from build123d import *

# Parameters (mm, degrees)
SKETCH1_R                    = 1.8288
BASE_FLANGE1_DEPTH           = 1.5875
EDGE_FLANGE2_STRIP_W         = 7.8232
EDGE_FLANGE2_STRIP_H         = 1.5875
EDGE_FLANGE2_STRIP_CUT_DEPTH = 6.35
EDGE_FLANGE2_DEPTH           = 6.35
SKETCH19_W                   = 5.65
SKETCH19_H                   = 12
TAB1_DEPTH                   = 1.5875
HOLE1_START                  = -28.75
HOLE1_OUTLINE_R              = 1.8288
HOLE1_DEPTH                  = 1.5875
FILLET1_R                    = 6


# Read off the part's stored shape, not the designer's step: Hole1
# Sheet-metal steps are written as plain solids
with BuildPart() as part:
    # Sketch1 → Base-Flange1 (new body)
    with BuildSketch(Plane(origin=(0, 0, 0), x_dir=(1, 0, 0), z_dir=(0, 1, 0))):
        with BuildLine():
            Line((-25.575, 0), (-25.575, 6.35))
            Line((-25.575, 6.35), (-27.1625, 6.35))
            Line((-27.1625, 6.35), (-27.1625, 12.7))
            Line((-27.1625, 12.7), (0, 12.7))
            Line((0, 12.7), (25.575, 12.7))
            Line((25.575, 12.7), (25.575, 0))
            ThreePointArc((25.575, 0), (22.4, -3.175), (19.225, 0))
            Line((19.225, 0), (19.225, 6.35))
            Line((19.225, 6.35), (3.175, 6.35))
            Line((3.175, 6.35), (3.175, 0))
            ThreePointArc((3.175, 0), (0, -3.175), (-3.175, 0))
            Line((-3.175, 0), (-3.175, 6.35))
            Line((-3.175, 6.35), (-19.225, 6.35))
            Line((-19.225, 6.35), (-19.225, 0))
            ThreePointArc((-19.225, 0), (-22.4, -3.175), (-25.575, 0))
        make_face()
        with Locations(Location((0, 0, 0), (0, 0, 270))):
            Circle(SKETCH1_R, mode=Mode.SUBTRACT)
        with Locations(Location((22.4, 0, 0), (0, 0, 270))):
            Circle(SKETCH1_R, mode=Mode.SUBTRACT)
        with Locations(Location((-22.4, 0, 0), (0, 0, 270))):
            Circle(SKETCH1_R, mode=Mode.SUBTRACT)
    extrude(amount=BASE_FLANGE1_DEPTH)

    # Edge-Flange2 strip (across the edge) → Edge-Flange2 strip cut (cut)
    with BuildSketch(Plane(origin=(-27.1625, 1.5875, -12.7), x_dir=(1, 0, 0), z_dir=(0, 0, 1))):
        with Locations((-3.175, -0.79375)):
            Rectangle(EDGE_FLANGE2_STRIP_W, EDGE_FLANGE2_STRIP_H)
    extrude(amount=EDGE_FLANGE2_STRIP_CUT_DEPTH, mode=Mode.SUBTRACT)

    # Edge-Flange2 section (across the edge) → Edge-Flange2 (add)
    with BuildSketch(Plane(origin=(-27.1625, 1.5875, -12.7), x_dir=(1, 0, 0), z_dir=(0, 0, 1))):
        with BuildLine():
            Line((-1.5875, 0.7366), (-1.5875, 31.688))
            Line((-1.5875, 31.688), (0, 31.688))
            Line((0, 31.688), (0, 0.7366))
            ThreePointArc((0, 0.7366), (0.215745145, 0.215745145), (0.7366, 0))
            Line((0.7366, 0), (0.7366, -1.5875))
            ThreePointArc((0.7366, -1.5875), (-0.90678687, -0.90678687), (-1.5875, 0.7366))
        make_face()
    extrude(amount=EDGE_FLANGE2_DEPTH)

    # Sketch19 → Tab1 (add)
    with BuildSketch(Plane.ZY.offset(28.75)):
        with Locations((-3.525, 27.2755)):
            Rectangle(SKETCH19_W, SKETCH19_H)
    extrude(amount=-TAB1_DEPTH)

    # Hole1 outline → Hole1 (cut)
    with BuildSketch(Plane.YZ.offset(HOLE1_START)):
        with Locations((26.9255, -6.7)):
            Circle(HOLE1_OUTLINE_R)
    extrude(amount=HOLE1_DEPTH, mode=Mode.SUBTRACT)

    # Fillet1
    # the kernel refuses this fillet: 6 mm, written as the material it takes off along each edge
    with BuildSketch(Plane(origin=(-43.724457419, 21.2755, -0.7), x_dir=(0, 0, -1), z_dir=(1, 0, 0))) as fillet1_piece_1:
        with BuildLine():
            CenterArc((6, 5.989782968), FILLET1_R, 180, 86.655847796)
            Line((0, 5.989782968), (-0.12, 5.989782968))
            Line((-0.12, 5.989782968), (-0.12, 0))
            Line((-0.12, 0), (0, -0.12))
            ThreePointArc((0, -0.12), (2.825, -0.12), (5.643, -0.119795659))
            Line((5.643, -0.119795659), (5.65, 0))
        make_face()
    extrude(amount=31.536414838, mode=Mode.SUBTRACT)
    with BuildSketch(Plane(origin=(-43.75, 33.2755, -0.7), x_dir=(0, 0, -1), z_dir=(1, 0, 0)), Plane(origin=(-43.75, 33.2755, -12.7), x_dir=(0, -1, 0), z_dir=(1, 0, 0))) as fillet1_piece_2:
        with BuildLine():
            CenterArc((FILLET1_R, -FILLET1_R), FILLET1_R, 90, 90)
            Line((0, -FILLET1_R), (-FILLET1_R * 0.02, -FILLET1_R))
            Line((-FILLET1_R * 0.02, -FILLET1_R), (-FILLET1_R * 0.02, FILLET1_R * 0.02))
            Line((-FILLET1_R * 0.02, FILLET1_R * 0.02), (FILLET1_R, FILLET1_R * 0.02))
            Line((FILLET1_R, FILLET1_R * 0.02), (FILLET1_R, 0))
        make_face()
    extrude(amount=31.5875, mode=Mode.SUBTRACT)


solid = part.part
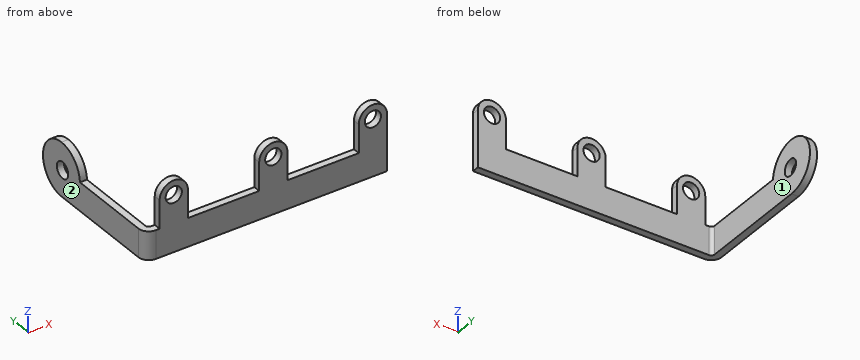
Part model, mm, in its own coordinate system. Face numbers are marked on the shaded views. A direction names the side the tool comes from. Coordinates: 2 decimals unless noted, no trailing zeros. Order: outer loops, then holes, each group sorted by start corner. A loop starts at its lowest first (then second) coordinate and runs counter-clockwise, first axis right, second up. Notation, with made-up numbers: (-10, -24.75) - (45, -24.75) arc R18 ccw to (45, -7.75) - close; hole circle Ø7 at (55, 9). An arc over 180 degrees is marked (long way). Use CSV: the item, a comma, the result in double quotes.
Item 1: Saw through at B-B on z = -4. Give the number of separate pieces and of enclosed holes in the cut face, and give its area (3 significant figures).
Solved:
separate pieces,"4"
enclosed holes,"0"
area,"47.3 mm²"
Item 2: 3-axis set-ups, long thin cutter, end or side, ignore diameter. For the marked faces 1 and 2: which of +Z, -Z, +X, -X, +Y, -Y reach the whole face in a straight line?
Solved:
face 1,"+Z, -Z, +X, +Y"
face 2,"+Z, -Z, -X, +Y, -Y"
Item 3: Saw through at C-C on x = 7. Give the cut face in (y, z), and give its area (3 significant figures).
Solved:
outline,"(0, -12.7) - (1.59, -12.7) - (1.59, -6.35) - (0, -6.35) - close"
area,"10.1 mm²"
Item 4: Probe probe 1 along X at (y, z) = (28, -1); probe 2 along Y at (x, z) = (21, -12). List the from-to ranges inside material, lowest first.
Solved:
probe 1,"x = -28.75 to -27.16"
probe 2,"y = 0 to 1.59"
Item 5: Drop flat-ended pins along their axis: P1, Ø9.5, axis at y = 24.5, z = -5.5, coming from the +X side; P2, Ø3.5, axis at x = -26.5, y = 11, coming from the +Z side; P3, Ø0.5, axis at y = 0.5, z = -3.5, coming from the -X side (3 decimals). Give the stop position or say it passes through.
Solved:
P1,"stops at x = -27.16"
P2,"stops at z = -6.35"
P3,"stops at x = -25.575"
Item 6: Saw through at D-D on y = 19. Give the cut face in (x, z), and give its area (3 significant figures).
Solved:
outline,"(-28.75, -12.7) - (-27.16, -12.7) - (-27.16, -6.35) - (-28.75, -6.35) - close"
area,"10.1 mm²"
Item 7: Saw through at A-A on x = 0. Give the cut face in (y, z) (1 decimal), and give its area (3 significant figures).
Solved:
outline,"(0, -12.7) - (1.6, -12.7) - (1.6, -1.8) - (0, -1.8) - close; (0, 1.8) - (1.6, 1.8) - (1.6, 3.2) - (0, 3.2) - close"
area,"19.4 mm²"
